Part print with two shaded views. Sizes in mm from the minimum x, y, z corner. A direction names the side the tool comes from. Give positions to 0.01 mm unless a question says otherwise; leave off trailing zeros. Write each loop counter-clockwise with the first axis right and the second up, starting at its lowest first coordinate (ties: lowest second). Pieces come first, ordered by that corner, then holes.
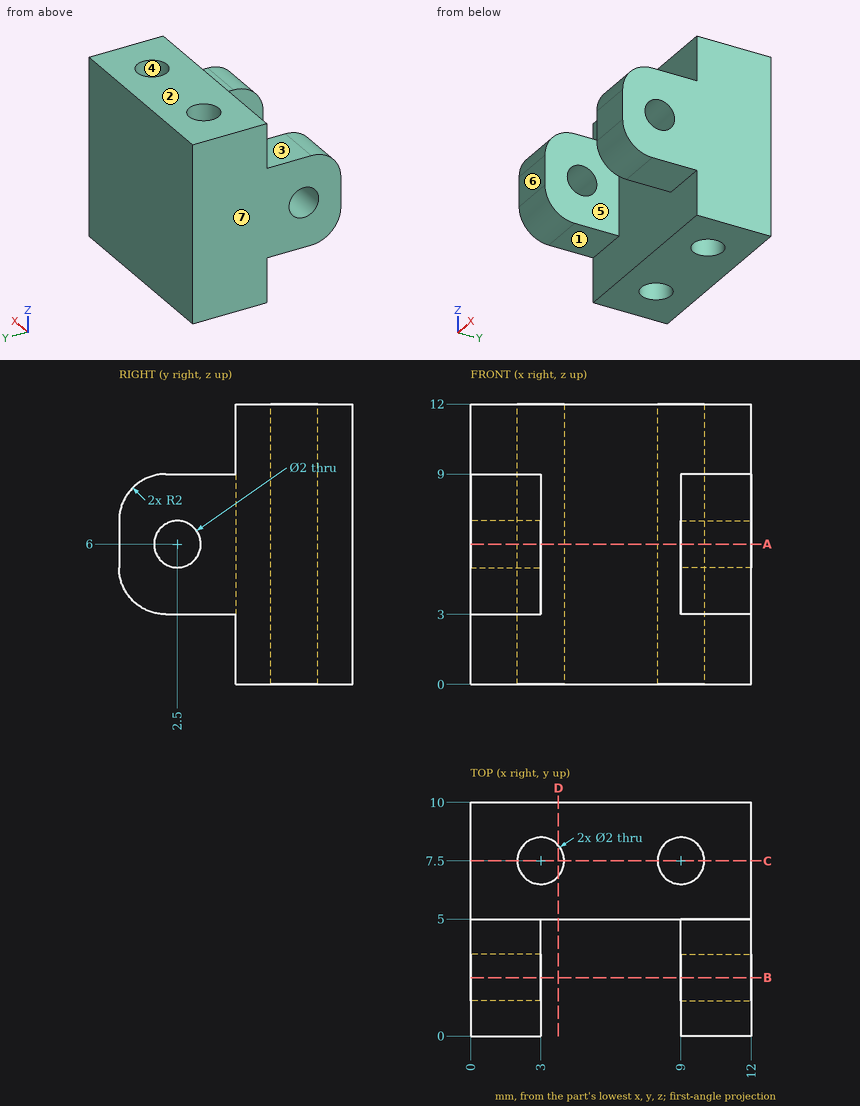
1) Two-plate mould, pull along X, no slides. Class the marked faces 4, 5, 6 and 7: +X half, -X half, draft (parallel to the pull), parting line (faces both ways), or undercut.
Answers follow:
face 4: undercut
face 5: undercut
face 6: draft
face 7: -X half
2) Saw through at B-B, the plane y = 2.5. Write the cut outline in (x, z).
Answers follow:
outline: (0, 3) - (3, 3) - (3, 5) - (0, 5) - close; (0, 7) - (3, 7) - (3, 9) - (0, 9) - close; (9, 3) - (12, 3) - (12, 5) - (9, 5) - close; (9, 7) - (12, 7) - (12, 9) - (9, 9) - close
3) Pin check, flat tips, straight feed: pin 1 Ø3.5 at (x, y) = (1, 3) entering from -Z; pin 2 Ø1.5 at (x, y) = (2, 3.5) entering from +Z. Stop position of each tip, or through.
Answers follow:
pin 1: stops at z = 3
pin 2: stops at z = 9
4) Saw through at D-D, the plane x = 3.75. Write the cut outline in (y, z), then the cut area to 3 significant figures.
Answers follow:
outline: (5, 0) - (6.84, 0) - (6.84, 12) - (5, 12) - close; (8.16, 0) - (10, 0) - (10, 12) - (8.16, 12) - close
area: 44.1 mm2
5) Saw through at A-A, the plane z = 6. Write the cut outline in (x, y), then the cut area to 3 significant figures.
Answers follow:
outline: (0, 0) - (3, 0) - (3, 1.5) - (0, 1.5) - close; (0, 3.5) - (3, 3.5) - (3, 5) - (9, 5) - (9, 3.5) - (12, 3.5) - (12, 10) - (0, 10) - close; (9, 0) - (12, 0) - (12, 1.5) - (9, 1.5) - close; hole circle Ø2 at (3, 7.5); hole circle Ø2 at (9, 7.5)
area: 71.7 mm2
6) Saw through at C-C, the plane y = 7.5. Write the cut outline in (x, z).
Answers follow:
outline: (0, 0) - (2, 0) - (2, 12) - (0, 12) - close; (4, 0) - (8, 0) - (8, 12) - (4, 12) - close; (10, 0) - (12, 0) - (12, 12) - (10, 12) - close
7) Wall check: L1, parallel to X at y = 2.5, z = 4.25; L2, parallel to Y at x = 11.2, z = 6; L3, parallel to X at y = 8.25, z = 6. Give the ranges that are in metal, low to high.
Answers follow:
L1: x = 0 to 3, 9 to 12
L2: y = 0 to 1.5, 3.5 to 10
L3: x = 0 to 2.34, 3.66 to 8.34, 9.66 to 12
8) 3-axis set-ups, long thin cutter, end or side, ignore diameter. For the marked faces 1, 2 and 3: which of +Z, -Z, +X, -X, +Y, -Y reach the whole face in a straight line?
Answers follow:
face 1: -Z, +X, -X, -Y
face 2: +Z, +X, -X, +Y, -Y
face 3: +Z, +X, -X, -Y
